Here's the drawing with two shaded views (mm, measured from the low corner). I have some questions. A direction names the side the tool comes from. Coordinates: 2 decimals unless noted, no trailing zeros. Loops run counter-clockwise (first coordinate to the right, second up) from the corner with the lowest first, then second, coordinate; pieces in that order, holes last. Notation, with made-up numbers: (-23.75, 19.25) - (21.25, 19.25) arc R38 ccw to (21.25, 57.25) - close; hole circle Ø9 at (-18, 67). An arc over 180 degrees is marked (long way). Use a Markdown table: item, result.
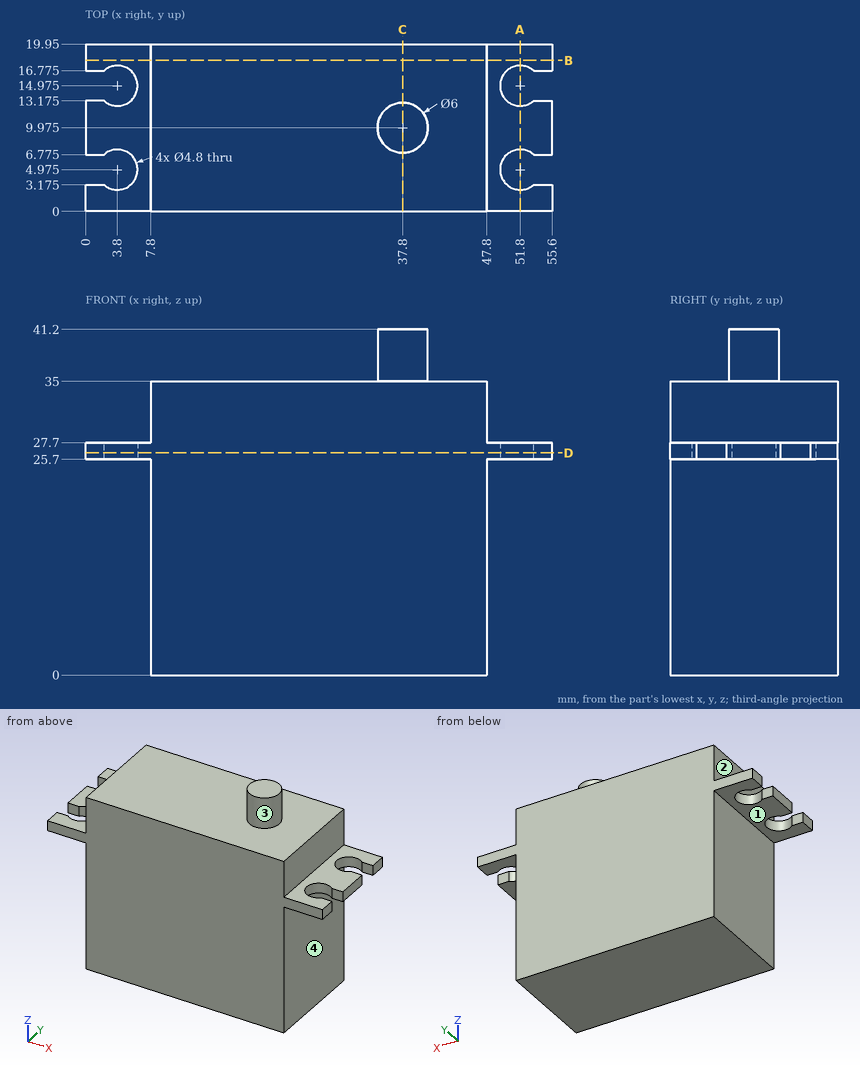
Q1. I want a section at B-B, the plane y = 18. Write out the boundary of the cut face in (x, z), then the cut area to 3 significant figures.
Check values:
| item | result |
|---|---|
| outline | (0, 25.7) - (7.8, 25.7) - (7.8, 0) - (47.8, 0) - (47.8, 25.7) - (55.6, 25.7) - (55.6, 27.7) - (47.8, 27.7) - (47.8, 35) - (7.8, 35) - (7.8, 27.7) - (0, 27.7) - close |
| area | 1,430 mm^2 |
Q2. I want a section at C-C, the plane x = 37.8. Write out the boundary of the cut face in (y, z) (3 decimals).
Check values:
| item | result |
|---|---|
| outline | (0, 0) - (19.95, 0) - (19.95, 35) - (12.975, 35) - (12.975, 41.2) - (6.975, 41.2) - (6.975, 35) - (0, 35) - close |
Q3. Which directions (+Z, -Z, +X, -X, +Y, -Y) give clear straight access to the entire face, cutting with the end or side of a thin tool? Please do the marked faces 1, 2, 3 and 4.
Check values:
| item | result |
|---|---|
| face 1 | -Z, -X, +Y, -Y |
| face 2 | +Z, -X, +Y, -Y |
| face 3 | +Z |
| face 4 | -Z, +X, +Y, -Y |
Q4. Please list where these lines run through material, in increasing order: L1, parallel to Y at x = 51.8, z = 27.05 (3 decimals); L2, parallel to Y at x = 51, z = 27; L3, parallel to Z at x = 43, y = 18.5. Write a range as from..to.
Check values:
| item | result |
|---|---|
| L1 | 0..2.575, 7.375..12.575, 17.375..19.95 |
| L2 | 0..2.71, 7.24..12.71, 17.24..19.95 |
| L3 | 0..35 |
Q5. I want a section at A-A, the plane x = 51.8. Write out the boundary of the cut face in (y, z) (3 decimals).
Check values:
| item | result |
|---|---|
| outline | (0, 25.7) - (2.575, 25.7) - (2.575, 27.7) - (0, 27.7) - close; (7.375, 25.7) - (12.575, 25.7) - (12.575, 27.7) - (7.375, 27.7) - close; (17.375, 25.7) - (19.95, 25.7) - (19.95, 27.7) - (17.375, 27.7) - close |
Q6. Will these pins go through, and if not, where does the flat tip stop? P1, Ø6, axis at x = 3.5, y = 12, coming from the -Z side; P2, Ø8.5, axis at x = 50.5, y = 12.5, coming from the +Z side; P3, Ø1.5, axis at y = 16.5, z = 9, coming from the +X side.
Check values:
| item | result |
|---|---|
| P1 | z = 25.7 |
| P2 | z = 35 |
| P3 | x = 47.8 |
Q7. I want a section at D-D, the plane z = 26.5. Write out the boundary of the cut face in (x, y) (3 decimals).
Check values:
| item | result |
|---|---|
| outline | (0, 0) - (55.6, 0) - (55.6, 3.175) - (53.387, 3.175) arc R2.4 cw (long way) to (53.387, 6.775) - (55.6, 6.775) - (55.6, 13.175) - (53.387, 13.175) arc R2.4 cw (long way) to (53.387, 16.775) - (55.6, 16.775) - (55.6, 19.95) - (0, 19.95) - (0, 16.775) - (2.213, 16.775) arc R2.4 cw (long way) to (2.213, 13.175) - (0, 13.175) - (0, 6.775) - (2.213, 6.775) arc R2.4 cw (long way) to (2.213, 3.175) - (0, 3.175) - close |
